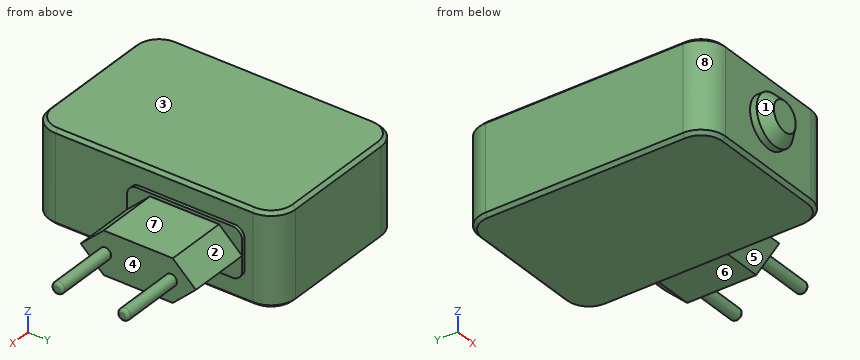
from build123d import *

# Parameters (mm, degrees)
SKETCH_W        = 50
SKETCH_H        = 75
PAD_DEPTH       = 14
FILLET_R        = 7.5
CHAMFER_SIZE    = 1
SKETCH001_W     = 35
SKETCH001_H     = 15
PAD001_DEPTH    = 1
FILLET001_R     = 3
PAD002_DEPTH    = 19
SKETCH003_R     = 1.75
PAD003_DEPTH    = 20
FILLET002_R     = 1
SKETCH004_R     = 7.5
PAD004_DEPTH    = 1.5
SKETCH005_R     = 7.5
PAD005_DEPTH    = 3.5
CHAMFER001_SIZE = 3


with BuildPart() as part:
    # Sketch → Pad (new body, symmetric)
    with BuildSketch(Plane.XY):
        Rectangle(SKETCH_W, SKETCH_H)
    extrude(amount=PAD_DEPTH, both=True)

    # Fillet
    fillet_edges = [part.edges().sort_by_distance(p)[0] for p in [
        (25, -37.5, 0),
        (-25, -37.5, 0),
        (25, 37.5, 0),
        (-25, 37.5, 0),
    ]]
    fillet(fillet_edges, radius=FILLET_R)

    # Chamfer
    chamfer_edges = [part.edges().sort_by_distance(p)[0] for p in [
        (0, 37.5, 14),
        (-22.803301, 35.303301, 14),
        (-25, 0, 14),
        (25, 0, 14),
        (22.803301, 35.303301, 14),
        (-22.803301, -35.303301, 14),
        (0, -37.5, 14),
        (22.803301, -35.303301, 14),
        (22.803301, -35.303301, -14),
        (0, -37.5, -14),
        (-22.803301, -35.303301, -14),
        (-25, 0, -14),
        (25, 0, -14),
        (22.803301, 35.303301, -14),
        (0, 37.5, -14),
        (-22.803301, 35.303301, -14),
    ]]
    chamfer(chamfer_edges, length=CHAMFER_SIZE)

    # Sketch001 (on Face13 of Chamfer) → Pad001 (join)
    with BuildSketch(Plane.YZ.offset(25)):
        with Locations((10, 0)):
            Rectangle(SKETCH001_W, SKETCH001_H)
    extrude(amount=PAD001_DEPTH)

    # Fillet001
    fillet001_edges = [part.edges().sort_by_distance(p)[0] for p in [
        (25.5, 27.5, 7.5),
        (25.5, 27.5, -7.5),
        (25.5, -7.5, -7.5),
        (25.5, -7.5, 7.5),
    ]]
    fillet(fillet001_edges, radius=FILLET001_R)

    # Sketch002 (on Face14 of Fillet001) → Pad002 (join)
    with BuildSketch(Plane.YZ.offset(26)):
        Polygon((27.5, 0), (20.5, 6.5), (-0.5, 6.5), (-7.5, 0), (-0.5, -6.5), (20.5, -6.5), align=None)
    extrude(amount=PAD002_DEPTH)

    # Sketch003 (on Face42 of Pad002) → Pad003 (join)
    with BuildSketch(Plane.YZ.offset(45)):
        Circle(SKETCH003_R)
        with Locations((20, 0)):
            Circle(SKETCH003_R)
    extrude(amount=PAD003_DEPTH)

    # Fillet002
    fillet002_edges = [part.edges().sort_by_distance(p)[0] for p in [
        (65, -1.75, 0),
        (65, 18.25, 0),
    ]]
    fillet(fillet002_edges, radius=FILLET002_R)

    # Sketch004 (on Face36 of Fillet002) → Pad004 (join)
    with BuildSketch(Plane.XZ.offset(37.5)):
        Circle(SKETCH004_R)
    extrude(amount=PAD004_DEPTH)

    # Sketch005 (on Face51 of Pad004) → Pad005 (join)
    with BuildSketch(Plane.XZ.offset(39)):
        Circle(SKETCH005_R)
    extrude(amount=PAD005_DEPTH)

    # Chamfer001
    chamfer001_edges = [part.edges().sort_by_distance(p)[0] for p in [
        (-7.5, -42.5, 0),
    ]]
    chamfer(chamfer001_edges, length=CHAMFER001_SIZE)


solid = part.part
The listing builds one solid part. Answer for the finished solid, in the listing's coordinates (mm). Face numbers are marked on the shaded views. A direction names the side the tool comes from. Give positions to 0.01 mm unless a question says otherwise; leave off trailing zeros. Loops run counter-clockwise (first coordinate to the right, second up) from the corner with the lowest first, then second, coordinate; pieces in that order, holes last. Notation, with made-up numbers: M -22.5,-33 L 14.5,-33 A18 cw 14.5,-18 Z; hole C 65.25,51.5 d11. An arc over 180 degrees is marked long. Answer as CSV lines item,"result".
Item 1: The part is cut by section D-D (x = 0). Give the vertices of the cut face in (y, z), and give its area (3 significant figures).
Values follow:
outline,"M -42.5,-4.5 L -39.5,-7.5 L -37.5,-7.5 L -37.5,-13 L -36.5,-14 L 36.5,-14 L 37.5,-13 L 37.5,13 L 36.5,14 L -36.5,14 L -37.5,13 L -37.5,7.5 L -39.5,7.5 L -42.5,4.5 Z"
area,"2,160 mm^2"
Item 2: Which of the six approach directions +Z, -Z, +X, -X, +Y, -Y give full straight-line access (tool end or side, diameter ignored) to the marked faces 5, 6, 7 and 8?
Values follow:
face 5,"-Z, +X, -Y"
face 6,"-Z, +X, +Y, -Y"
face 7,"+Z, +X, +Y, -Y"
face 8,"+Z, -Z, -X, -Y"
Item 3: The part is cut by section A-A (y = 11). Give the vertices of the cut face in (x, z), and give its area (3 significant figures).
Values follow:
outline,"M -25,-13 L -24,-14 L 24,-14 L 25,-13 L 25,-7.5 L 26,-7.5 L 26,-6.5 L 45,-6.5 L 45,6.5 L 26,6.5 L 26,7.5 L 25,7.5 L 25,13 L 24,14 L -24,14 L -25,13 Z"
area,"1,660 mm^2"
Item 4: The mould has two halves that part along Y. Classify the marked faces 1, 2, 3 and 4: released by +Y, released by -Y, zero draft, split by the parting line, or undercut.
Values follow:
face 1,"released by -Y"
face 2,"released by +Y"
face 3,"zero draft"
face 4,"undercut"
Item 5: Given pin 1 Ø0.5 at (x, y) = (25.5, 15.5) entering from +Z; pin 2 Ø21 at (x, y) = (38, 12.5) entering from -Z; pin 3 Ø0.8 at (x, z) = (25.5, 2) entering from +Y; pin 4 Ø10.5 at (y, z) = (17.5, 3) entering from +X, each flat-ended and moving along its own axis, determine where each tip first touches the part or whether it passes through.
Values follow:
pin 1,"stops at z = 7.5"
pin 2,"stops at z = -6.5"
pin 3,"stops at y = 27.5"
pin 4,"stops at x = 65"
Item 6: The part is cut by section C-C (x = 14). Give the vertices of the cut face in (y, z), and give its area (3 significant figures).
Values follow:
outline,"M -37.5,-13 L -36.5,-14 L 36.5,-14 L 37.5,-13 L 37.5,13 L 36.5,14 L -36.5,14 L -37.5,13 Z"
area,"2,100 mm^2"
Item 7: Straight lines are drawn through the part: line 1 along X through (y, z) = (18, 10); line 2 along Z through (x, y) = (42, 12.5); line 3 along Y through (x, z) = (-18, -8.75). For each, find the intervals that lie inside material, in ascending order. Write a range as [from, to].
Values follow:
line 1,"x = [-25, 25]"
line 2,"z = [-6.5, 6.5]"
line 3,"y = [-37.48, 37.48]"
Item 8: The part is cut by section B-B (z = 8.5). Give the vertices of the cut face in (x, y), and give its area (3 significant figures).
Values follow:
outline,"M -25,-30 A7.5 ccw -17.5,-37.5 L 17.5,-37.5 A7.5 ccw 25,-30 L 25,30 A7.5 ccw 17.5,37.5 L -17.5,37.5 A7.5 ccw -25,30 Z"
area,"3,700 mm^2"
